Geometry check sheet. Reference: the model listing, model coordinates, mm. Round coordinates to 2 decimals unless told otherwise and drop trailing zeros. Write each loop counter-clockwise with the first axis right and the second up, starting at its lowest first coordinate (ties: lowest second). Pieces come first, ordered by that corner, then holes. Notation, with made-up numbers: M 27,81 L 81,81 A19 ccw 81,94 Z; hole C -7,-20 d5. An arc over 180 degrees is marked long. Use a Markdown table: item, result.
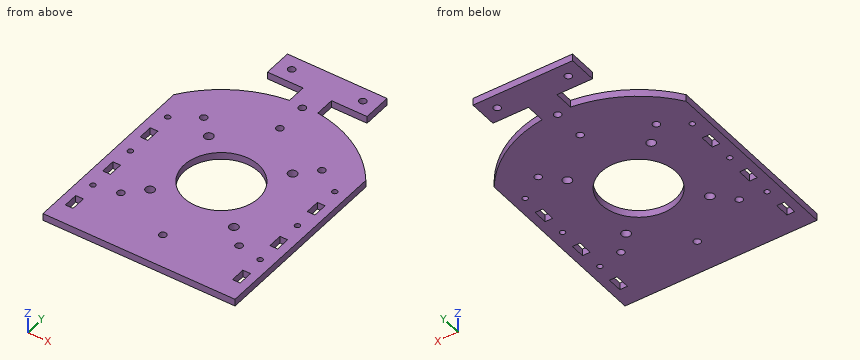
```python
from build123d import *

# Parameters (mm, degrees)
SKETCH_1_R      = 1.5
SKETCH_1_R_2    = 2.5
SKETCH_1_R_3    = 21
SKETCH_1_R_4    = 2
SKETCH_1_W      = 4.3
SKETCH_1_H      = 8.1
SKETCH_1_H_2    = 8.3
EXTRUDE_1_DEPTH = 4


with BuildPart() as part:
    # 草图1 → 凸台-拉伸1 (new body)
    with BuildSketch(Plane.XY):
        with BuildLine():
            Line((-54, 52.4), (-54, -52.6))
            Line((-54, -52.6), (54, -52.6))
            Line((54, -52.6), (54, 52.4))
            ThreePointArc((54, 52.4), (33.845954515, 70.803240423), (8, 79.569735886))
            Line((8, 79.569735886), (8, 90.5))
            Line((8, 90.5), (28, 90.5))
            Line((28, 90.5), (28, 106.5))
            Line((28, 106.5), (-28, 106.5))
            Line((-28, 106.5), (-28, 90.5))
            Line((-28, 90.5), (-8, 90.5))
            Line((-8, 90.5), (-8, 79.569735886))
            ThreePointArc((-8, 79.569735886), (-33.845954515, 70.803240423), (-54, 52.4))
        make_face()
        with Locations((-47, 37.5)):
            Circle(SKETCH_1_R, mode=Mode.SUBTRACT)
        with Locations((-47, 7.5)):
            Circle(SKETCH_1_R, mode=Mode.SUBTRACT)
        with Locations((-47, -22.5)):
            Circle(SKETCH_1_R, mode=Mode.SUBTRACT)
        with Locations((-23.57, 37.07)):
            Circle(SKETCH_1_R_2, mode=Mode.SUBTRACT)
        with Locations((-23.57, -10.07)):
            Circle(SKETCH_1_R_2, mode=Mode.SUBTRACT)
        with Locations((23.57, -10.07)):
            Circle(SKETCH_1_R_2, mode=Mode.SUBTRACT)
        with Locations((23.57, 37.07)):
            Circle(SKETCH_1_R_2, mode=Mode.SUBTRACT)
        with Locations((47, -22.5)):
            Circle(SKETCH_1_R, mode=Mode.SUBTRACT)
        with Locations((47, 7.5)):
            Circle(SKETCH_1_R, mode=Mode.SUBTRACT)
        with Locations((47, 37.5)):
            Circle(SKETCH_1_R, mode=Mode.SUBTRACT)
        with Locations((0, 13.5)):
            Circle(SKETCH_1_R_3, mode=Mode.SUBTRACT)
        with Locations((0, 60.5)):
            Circle(SKETCH_1_R_4, mode=Mode.SUBTRACT)
        with Locations((33.234018716, 46.734018716)):
            Circle(SKETCH_1_R_4, mode=Mode.SUBTRACT)
        with Locations((33.234018716, -19.734018716)):
            Circle(SKETCH_1_R_4, mode=Mode.SUBTRACT)
        with Locations((0, -33.5)):
            Circle(SKETCH_1_R_4, mode=Mode.SUBTRACT)
        with Locations((-33.234018716, -19.734018716)):
            Circle(SKETCH_1_R_4, mode=Mode.SUBTRACT)
        with Locations((-33.234018716, 46.734018716)):
            Circle(SKETCH_1_R_4, mode=Mode.SUBTRACT)
        with Locations((0, 78.5)):
            Circle(SKETCH_1_R_4, mode=Mode.SUBTRACT)
        with Locations((-20, 98.5)):
            Circle(SKETCH_1_R_4, mode=Mode.SUBTRACT)
        with Locations((20, 98.5)):
            Circle(SKETCH_1_R_4, mode=Mode.SUBTRACT)
        with Locations((-47, 22.5)):
            Rectangle(SKETCH_1_W, SKETCH_1_H, mode=Mode.SUBTRACT)
        with Locations((-47, -7.5)):
            Rectangle(SKETCH_1_W, SKETCH_1_H, mode=Mode.SUBTRACT)
        with Locations((-47, -37.4)):
            Rectangle(SKETCH_1_W, SKETCH_1_H_2, mode=Mode.SUBTRACT)
        with Locations((47, -37.4)):
            Rectangle(SKETCH_1_W, SKETCH_1_H_2, mode=Mode.SUBTRACT)
        with Locations((47, -7.5)):
            Rectangle(SKETCH_1_W, SKETCH_1_H, mode=Mode.SUBTRACT)
        with Locations((47, 22.5)):
            Rectangle(SKETCH_1_W, SKETCH_1_H, mode=Mode.SUBTRACT)
    extrude(amount=EXTRUDE_1_DEPTH)


solid = part.part
```
Item 1: Material ranges on line 1 along Y through (x, z) = (0, 1.45); line 2 along Y through (x, z) = (-8.5, 2.5); line 3 along Y through (x, z) = (13.5, 1.95), recorded low to high. Write a range as from..to.
Outcome:
| item | result |
|---|---|
| line 1 | y = -52.6..-35.5, -31.5..-7.5, 34.5..58.5, 62.5..76.5, 80.5..106.5 |
| line 2 | y = -52.6..-5.7, 32.7..79.51, 90.5..106.5 |
| line 3 | y = -52.6..-2.59, 29.59..78.67, 90.5..106.5 |
Item 2: Cross-section at C-C, the plane x = -33. Record the cut outline in (y, z).
Outcome:
| item | result |
|---|---|
| outline | M -52.6,0 L -21.72,0 L -21.72,4 L -52.6,4 Z; M -17.75,0 L 44.75,0 L 44.75,4 L -17.75,4 Z; M 48.72,0 L 71.29,0 L 71.29,4 L 48.72,4 Z |
Item 3: Cross-section at A-A, the plane x = 0. Record the cut outline in (y, z).
Outcome:
| item | result |
|---|---|
| outline | M -52.6,0 L -35.5,0 L -35.5,4 L -52.6,4 Z; M -31.5,0 L -7.5,0 L -7.5,4 L -31.5,4 Z; M 34.5,0 L 58.5,0 L 58.5,4 L 34.5,4 Z; M 62.5,0 L 76.5,0 L 76.5,4 L 62.5,4 Z; M 80.5,0 L 106.5,0 L 106.5,4 L 80.5,4 Z |
Item 4: Cross-section at D-D, the plane x = 23.57. Record the cut outline in (y, z), and give its area (3 significant figures).
Outcome:
| item | result |
|---|---|
| outline | M -52.6,0 L -12.57,0 L -12.57,4 L -52.6,4 Z; M -7.57,0 L 34.57,0 L 34.57,4 L -7.57,4 Z; M 39.57,0 L 75.74,0 L 75.74,4 L 39.57,4 Z; M 90.5,0 L 106.5,0 L 106.5,4 L 90.5,4 Z |
| area | 537 mm2 |
Item 5: Cross-section at B-B, the plane y = 60.5. Record the cut outline in (x, z).
Outcome:
| item | result |
|---|---|
| outline | M -47.12,0 L -2,0 L -2,4 L -47.12,4 Z; M 2,0 L 47.12,0 L 47.12,4 L 2,4 Z |
Item 6: Go/stop test with a flat-tipped pin: pin 1 (1.5 mm diameter, centred on y = 76, z = 3, fed in from +X). Record where the tip stops, or that it passes through.
Outcome:
| item | result |
|---|---|
| pin 1 | stops at x = 24.82 |
